Check sheet for the modelled part. Datum: model origin and axes. Units: mm. A direction names the side the tool comes from. Round coordinates to 2 decimals unless told otherwise and drop trailing zeros. Order: outer loops, then holes, each group sorted by start corner. A loop starts at its lowest first (then second) coordinate and runs counter-clockwise, first axis right, second up. Notation, with made-up numbers: (54.25, 84) -> (99.25, 84) arc R23 cw to (99.25, 118) -> close; hole circle Ø9 at (31, 77.5). An arc over 180 degrees is marked (long way). Answer in a Markdown table with one row per item.
```python
from build123d import *

# Parameters (mm, degrees)
F0_W      = 50.8
F0_H      = 50.8
F1_DEPTH  = 50.8
F2_T      = -2.54
F3_W      = 14.649291
F3_H      = 24.7973
F3_W_2    = 10.16
F3_H_2    = 10.16
F4_DEPTH  = 22.352
F6_DEPTH  = 50.8
F7_W      = 33.02
F7_H      = 12.7
F8_DEPTH  = 84.836
F9_R      = 4.354014
F10_DEPTH = 25.4


with BuildPart() as f1:
    # F0 (on Top) → F1 (new body)
    with BuildSketch(Plane.XY):
        with Locations((-1.426203, 2.702715)):
            Rectangle(F0_W, F0_H)
    extrude(amount=F1_DEPTH)

    # F2
    f2_openings = [f1.faces().sort_by_distance(p)[0] for p in [
        (-1.426203, 2.702715, 0),
    ]]
    offset(amount=F2_T, openings=f2_openings)

    # F3 (on face) → F4 (cut)
    with BuildSketch(Plane.XZ.offset(22.697285)):
        with Locations((-8.750849, 12.39865)):
            Rectangle(F3_W, F3_H)
        with Locations((9.98387, 20.866262)):
            Rectangle(F3_W_2, F3_H_2)
    extrude(amount=-F4_DEPTH, mode=Mode.SUBTRACT)

    # F5 (on face) → F6 (join)
    with BuildSketch(Plane.XZ.offset(22.697285)):
        Polygon((0, 68.315133), (-26.826203, 50.8), (23.973797, 50.8), align=None)
    extrude(amount=-F6_DEPTH)

    # F7 (on face) → F8 (cut)
    with BuildSketch(Plane.YZ.offset(23.973797)):
        with Locations((2.292057, 23.624347)):
            Rectangle(F7_W, F7_H)
    extrude(amount=-F8_DEPTH, mode=Mode.SUBTRACT)

    # F9 (on face) → F10 (cut)
    with BuildSketch(Plane.XZ.offset(22.697285)):
        with Locations((0, 56.335028)):
            Circle(F9_R)
    extrude(amount=-F10_DEPTH, mode=Mode.SUBTRACT)


solid = f1.part
```
(1) Tool access check on faces 4 (the flat face through (0, 2.703, 56)), 5 (the flat face through (23, 2, 17.274)), 6 (the flat face through (-2, 3, 48.26)). Record the directions out of +Z, -Z, +X, -X, +Y, -Y that give a thin tool (end or side, any length) a straight path to the whole face; none if there is none.
Solutions:
| item | result |
|---|---|
| face 4 | -Y |
| face 5 | +X, -X |
| face 6 | -Z |
(2) Section check B-B on y = 8.5. Record the boundary of the cut face in (x, z).
Solutions:
| item | result |
|---|---|
| outline | (-26.83, 0) -> (-24.29, 0) -> (-24.29, 17.27) -> (-26.83, 17.27) -> close; (-26.83, 29.97) -> (-24.29, 29.97) -> (-24.29, 48.26) -> (21.43, 48.26) -> (21.43, 29.97) -> (23.97, 29.97) -> (23.97, 50.8) -> (0, 68.32) -> (-26.83, 50.8) -> close; (21.43, 0) -> (23.97, 0) -> (23.97, 17.27) -> (21.43, 17.27) -> close |
(3) Section check C-C on x = -8. Record the boundary of the cut face in (y, z).
Solutions:
| item | result |
|---|---|
| outline | (-22.7, 24.8) -> (-20.16, 24.8) -> (-20.16, 48.26) -> (25.56, 48.26) -> (25.56, 0) -> (28.1, 0) -> (28.1, 63.09) -> (-22.7, 63.09) -> close |
(4) Draft check along Y on faces 1 (the flat face through (-1.426, -21, 12)), 2 (the flat face through (-2, -22.697, 35)), 3 (the flat face through (-26, 2, 29.974)). Enter one of: pulls with the +Y half, pulls with the -Y half, needs draft (parallel to the pull), parting line crosses it, or undercut.
Solutions:
| item | result |
|---|---|
| face 1 | needs draft |
| face 2 | pulls with the -Y half |
| face 3 | undercut |
(5) Section check D-D on z = 12. Record the boundary of the cut face in (x, y), plus the area to 3 significant figures.
Solutions:
| item | result |
|---|---|
| outline | (-26.83, -22.7) -> (-16.08, -22.7) -> (-16.08, -20.16) -> (-24.29, -20.16) -> (-24.29, 25.56) -> (21.43, 25.56) -> (21.43, -20.16) -> (-1.43, -20.16) -> (-1.43, -22.7) -> (23.97, -22.7) -> (23.97, 28.1) -> (-26.83, 28.1) -> close |
| area | 453 mm^2 |
(6) Scan lines: probe 1 along Y at (x, z) = (1, 5); probe 2 along X at (y, z) = (-18, 13); probe 3 along Y at (x, z) = (-24.5, 27). Record each from-to range of solid material in increasing order. Write a range as from..to.
Solutions:
| item | result |
|---|---|
| probe 1 | -22.7..-20.16, 25.56..28.1 |
| probe 2 | -26.83..-24.29, 21.43..23.97 |
| probe 3 | -22.7..-14.22, 18.8..28.1 |
(7) Section check A-A on z = 43. Record the boundary of the cut face in (x, y).
Solutions:
| item | result |
|---|---|
| outline | (-26.83, -22.7) -> (23.97, -22.7) -> (23.97, 28.1) -> (-26.83, 28.1) -> close; hole (-24.29, -20.16) -> (21.43, -20.16) -> (21.43, 25.56) -> (-24.29, 25.56) -> close |
(8) Depth check by flat-ended pin: pin 1 Ø2.5 at (x, z) = (-1.5, 55.5) entering from -Y; pin 2 Ø0.8 at (x, y) = (23, -2) entering from -Z; pin 3 Ø12 at (x, y) = (-8, -15.5) entering from +Z; pin 4 Ø3 at (x, y) = (22.5, 5) entering from +Z. Enter the tip coordinate at first touch or a pass-through.
Solutions:
| item | result |
|---|---|
| pin 1 | y = 2.7 |
| pin 2 | z = 0 |
| pin 3 | z = 67.01 |
| pin 4 | z = 52.97 |
